The model under review builds one solid part; all positions refer to its coordinate system, in mm. Round coordinates to 2 decimals unless told otherwise and drop trailing zeros. Write each loop counter-clockwise with the first axis right and the second up, starting at its lowest first coordinate (ties: lowest second). Pieces come first, ordered by that corner, then holes. Notation, with made-up numbers: M 50.5,1 L 79.5,1 A22 cw 79.5,40 Z; hole C 53.25,36.5 d3. An arc over 180 degrees is marked long. Write item = value, one per line. Start each with the question number.
Item 1: Take a section at A-A, the plane y = 0. Give the boundary of the cut face in (x, z).
Item 2: Take a section at D-D, the plane x = 24. Give the boundary of the cut face in (y, z).
Item 3: Take a section at B-B, the plane x = -2. Give the boundary of the cut face in (y, z).
Item 4: Take a section at C-C, the plane z = 0.05. Give the boundary of the cut face in (x, y), plus the area to 3 significant figures.
Item 5: To check wall thickness, follow line 1 along Y through (x, z) = (0, 0.15); line 2 along X through (y, z) = (-12.5, -0.1); line 3 along Y through (x, z) = (-7.5, 0.05). State the ranges of each line that lie inside material, in increasing order.
from build123d import *

# Parameters (mm, degrees)
SKETCH1_R           = 12.5
SKETCH1_R_2         = 5
BOSS_EXTRUDE2_DEPTH = 0.2
SCALE1_SCALE        = 1.9329
SCALE2_SCALE        = 1.5


with BuildPart() as part:
    # Sketch1 → Boss-Extrude2 (new body)
    with BuildSketch(Plane.XY):
        Circle(SKETCH1_R)
        Circle(SKETCH1_R_2, mode=Mode.SUBTRACT)
    extrude(amount=BOSS_EXTRUDE2_DEPTH)


with BuildPart() as part_1:
    # Scale1: scaled about (0, 0, 0.1)
    add(part.part.scale(SCALE1_SCALE).moved(Location((0, 0, -0.09329))))


with BuildPart() as part_2:
    # Scale2: scaled about (0, 0, 0.1)
    add(part_1.part.scale(SCALE2_SCALE).moved(Location((0, 0, -0.05))))


solid = part_2.part
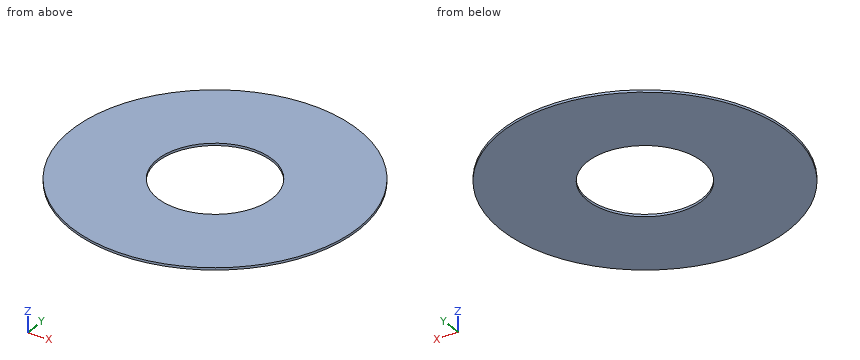
Response values:
q1.outline = M -36.24,-0.19 L -14.5,-0.19 L -14.5,0.39 L -36.24,0.39 Z; M 14.5,-0.19 L 36.24,-0.19 L 36.24,0.39 L 14.5,0.39 Z
q2.outline = M -27.16,-0.19 L 27.16,-0.19 L 27.16,0.39 L -27.16,0.39 Z
q3.outline = M -36.19,-0.19 L -14.36,-0.19 L -14.36,0.39 L -36.19,0.39 Z; M 14.36,-0.19 L 36.19,-0.19 L 36.19,0.39 L 14.36,0.39 Z
q4.outline = C 0,0 d72.48; hole C 0,0 d28.99
q4.area = 3,470 mm2
q5.line_1 = -36.24 to -14.5, 14.5 to 36.24
q5.line_2 = -34.02 to -7.34, 7.34 to 34.02
q5.line_3 = -35.46 to -12.41, 12.41 to 35.46
